from build123d import *

# Parameters (mm, degrees)
BOSS_EXTRUDE9_DEPTH   = 38.1
BOSS_EXTRUDE9_2_DEPTH = 38.1
BOSS_EXTRUDE10_DEPTH  = 50.8
SKETCH3_R             = 6.5532
CUT_EXTRUDE3_DEPTH    = 101.6


with BuildPart() as part:
    # Sketch1 → Boss-Extrude9 (new, symmetric)
    with BuildSketch(Plane.XY):
        with BuildLine():
            ThreePointArc((-76.2, -15.875), (-66.900640303, 6.575640303), (-44.45, 15.875))
            Line((-44.45, 15.875), (-88.9, 15.875))
            Line((-88.9, 15.875), (-88.9, -15.875))
            Line((-88.9, -15.875), (-76.2, -15.875))
        make_face()
    extrude(amount=BOSS_EXTRUDE9_DEPTH, both=True)



with BuildPart() as body_2:
    # Sketch1 → Boss-Extrude9 2 (new, symmetric)
    with BuildSketch(Plane.XY):
        with BuildLine():
            Line((76.2, -15.875), (88.9, -15.875))
            Line((88.9, -15.875), (88.9, 15.875))
            Line((88.9, 15.875), (44.45, 15.875))
            ThreePointArc((44.45, 15.875), (66.900640303, 6.575640303), (76.2, -15.875))
        make_face()
    extrude(amount=BOSS_EXTRUDE9_2_DEPTH, both=True)


with BuildPart() as part_1:
    add(part.part)

    add(body_2.part)  # Boss-Extrude10 merges body 2
    # Sketch1_11 → Boss-Extrude10 (add, symmetric)
    with BuildSketch(Plane.XY):
        with BuildLine():
            Line((63.5, -15.875), (76.2, -15.875))
            ThreePointArc((76.2, -15.875), (66.900640303, 6.575640303), (44.45, 15.875))
            Line((44.45, 15.875), (-44.45, 15.875))
            ThreePointArc((-44.45, 15.875), (-66.900640303, 6.575640303), (-76.2, -15.875))
            Line((-76.2, -15.875), (-63.5, -15.875))
            ThreePointArc((-63.5, -15.875), (-44.45, 3.175), (-25.4, -15.875))
            Line((-25.4, -15.875), (2.119780236, -15.875))
            Line((2.119780236, -15.875), (25.4, -15.875))
            ThreePointArc((25.4, -15.875), (44.45, 3.175), (63.5, -15.875))
        make_face()
    extrude(amount=BOSS_EXTRUDE10_DEPTH, both=True)

    # Sketch3 → Cut-Extrude3 (cut)
    with BuildSketch(Plane(origin=(0, 15.875, 0), x_dir=(1, 0, 0), z_dir=(0, 1, 0))):
        with Locations(Location((-76.2, 19.05, 0), (0, 0, 180))):
            Circle(SKETCH3_R)
        with Locations(Location((0, 38.1, 0), (0, 0, 180))):
            Circle(SKETCH3_R)
        with Locations(Location((76.2, 19.05, 0), (0, 0, 180))):
            Circle(SKETCH3_R)
        with Locations((76.2, -19.05)):
            Circle(SKETCH3_R)
        with Locations(Location((0, -38.1, 0), (0, 0, 90))):
            Circle(SKETCH3_R)
        with Locations(Location((-76.2, -19.05, 0), (0, 0, 180))):
            Circle(SKETCH3_R)
    extrude(amount=-CUT_EXTRUDE3_DEPTH, mode=Mode.SUBTRACT)


solid = part_1.part
Read the model definition and answer for the solid it produces. Units are mm, in the model's axes. A direction names the side the tool comes from. Give positions to 0.01 mm unless a question says otherwise; leave off trailing zeros. Loops run counter-clockwise (first coordinate to the right, second up) from the corner with the lowest first, then second, coordinate; pieces in that order, holes last. Notation, with made-up numbers: M 38.5,67.5 L 42.5,67.5 A24 ccw 42.5,102.5 Z; hole C 10,-15.5 d1. An arc over 180 degrees is marked long. Write each question's results on one line, items separated by ' | '.
1. Straight lines are drawn through the part: line 1 (X direction, y = 8, z = 19); line 2 (Z direction, x = 76.2, y = -5); line 3 (X direction, y = -14, z = 33). For each, find the intervals that lie inside material, in ascending order. Write a range as [from, to].
Values:
line 1: x = [-88.9, -82.75], [-69.65, 69.65], [82.75, 88.9] | line 2: z = [-38.1, -25.6], [-12.5, 12.5], [25.6, 38.1] | line 3: x = [-88.9, -63.41], [-25.49, -4.12], [4.12, 25.49], [63.41, 88.9]
2. A tool of negligible diameter and unlimited length cuts with its end or side. For faces 1 (the face through (-88.9, 0, 1)), 2 (the face through (-66.652, 6.821, 44.539)), 3 (the face through (67.146, 6.327, -44.361)), 4 (the face through (-79.224, 0.222, 13.236)), 5 (the face through (76, 4, 38.1)), from which of +Z, -Z, +X, -X, +Y, -Y can it reach the whole face along a straight path? Write none if from no direction.
Values:
face 1: +Z, -Z, -X, +Y, -Y | face 2: +Z, -X, +Y | face 3: -Z, +X, +Y | face 4: +Y, -Y | face 5: +Z, +X, +Y
3. Section C-C on y = -12 is taken. State how many separate pieces and enclosed holes the cut face has, plus the area to 3 significant figures.
Values:
separate pieces: 3 | enclosed holes: 6 | area: 9,020 mm^2
4. Given pin 1 (10.5 mm diameter, centred on x = 0, z = 38.1, fed in from +Y); pin 2 (17 mm diameter, centred on x = 76.2, z = -19.05, fed in from -Y) (3 decimals); pin 3 (6 mm diameter, centred on x = -49, z = -38, fed in from -Y) (3 decimals), each flat-ended and moving along its own axis, determine where each tip first touches the part or whether it passes through.
Values:
pin 1: passes through | pin 2: stops at y = -15.875 | pin 3: stops at y = 1.615
5. Section D-D on y = 12 is taken. Give the vertices of the cut face in (x, z).
Values:
outline: M -88.9,-38.1 L -59.65,-38.1 L -59.65,-50.8 L 59.65,-50.8 L 59.65,-38.1 L 88.9,-38.1 L 88.9,38.1 L 59.65,38.1 L 59.65,50.8 L -59.65,50.8 L -59.65,38.1 L -88.9,38.1 Z; hole C -76.2,-19.05 d13.11; hole C -76.2,19.05 d13.11; hole C 0,-38.1 d13.11; hole C 0,38.1 d13.11; hole C 76.2,-19.05 d13.11; hole C 76.2,19.05 d13.11
6. The mould has two halves that part along X. Classify faces 6 (the face through (-0.288, 0.222, 44.647)), 7 (the face through (88.9, 0, 1)), 8 (the face through (82.747, 0.222, -18.762)), 9 (the face through (-66.652, 6.821, -44.361)): pulls with the +X half, pulls with the -X half, needs draft (parallel to the pull), parting line crosses it, or undercut.
Values:
face 6: undercut | face 7: pulls with the +X half | face 8: undercut | face 9: pulls with the -X half
7. Section A-A on x = 0 is taken. Give the vertices of the cut face in (y, z) (3 decimals).
Values:
outline: M -15.875,-50.8 L 15.875,-50.8 L 15.875,-44.653 L -15.875,-44.653 Z; M -15.875,-31.547 L 15.875,-31.547 L 15.875,31.547 L -15.875,31.547 Z; M -15.875,44.653 L 15.875,44.653 L 15.875,50.8 L -15.875,50.8 Z
8. Section B-B on z = 19.05 is taken. Give the vertices of the cut face in (x, y) (3 decimals), plus the area to 3 significant figures.
Values:
outline: M -88.9,-15.875 L -82.753,-15.875 L -82.753,15.875 L -88.9,15.875 Z; M -69.647,-15.875 L -63.5,-15.875 A19.05 cw -25.4,-15.875 L 25.4,-15.875 A19.05 cw 63.5,-15.875 L 69.647,-15.875 L 69.647,15.875 L -69.647,15.875 Z; M 82.753,-15.875 L 88.9,-15.875 L 88.9,15.875 L 82.753,15.875 Z | area: 3,670 mm^2
